Here's the drawing with two shaded views (mm, measured from the low corner). I have some questions. A direction names the side the tool comes from. Coordinates: 2 decimals unless noted, no trailing zeros. Order: outer loops, then holes, each group sorted by start corner. A loop starts at its lowest first (then second) coordinate and runs counter-clockwise, first axis right, second up. Notation, with made-up numbers: (15, 11) - (40, 11) arc R30 cw to (40, 43) - close; hole circle Ø6 at (-36.75, 8.25). An arc over 180 degrees is marked (long way). Answer as a JSON object with one key per item and string values. Group by question number.
(1) Imagine slicing it at C-C, the plane y = 6.25. Write out the boundary of the cut face in (x, z).
(2) Imagine slicing it at B-B, the plane x = 3. Write out the boundary of the cut face in (y, z), and give its area (3 significant figures).
(3) Will this pin go through, and if not, where does the flat tip stop? P1, Ø1.5, axis at y = 6, z = 4, coming from the +X side.
(4) Which directions (+Z, -Z, +X, -X, +Y, -Y) give clear straight access to the entire face, cutting with the end or side of a thin tool? Please do the marked faces 1, 2 and 3.
(5) Please list where these lines run through material, in increasing order: probe 1 along Z at (x, y) = (3.5, 0.75); probe 2 along Y at (x, z) = (2.7, 3.9); probe 3 along Z at (x, y) = (5, 2.25).
(6) Imagine slicing it at A-A, the plane y = 0.75. Write out the boundary of the cut face in (x, z).
(7) We'd pull the mould along Z, two halves only. Please class the marked faces 4, 5 and 6: pulls with the +Z half, pulls with the -Z half, needs draft (parallel to the pull), parting line crosses it, or undercut.
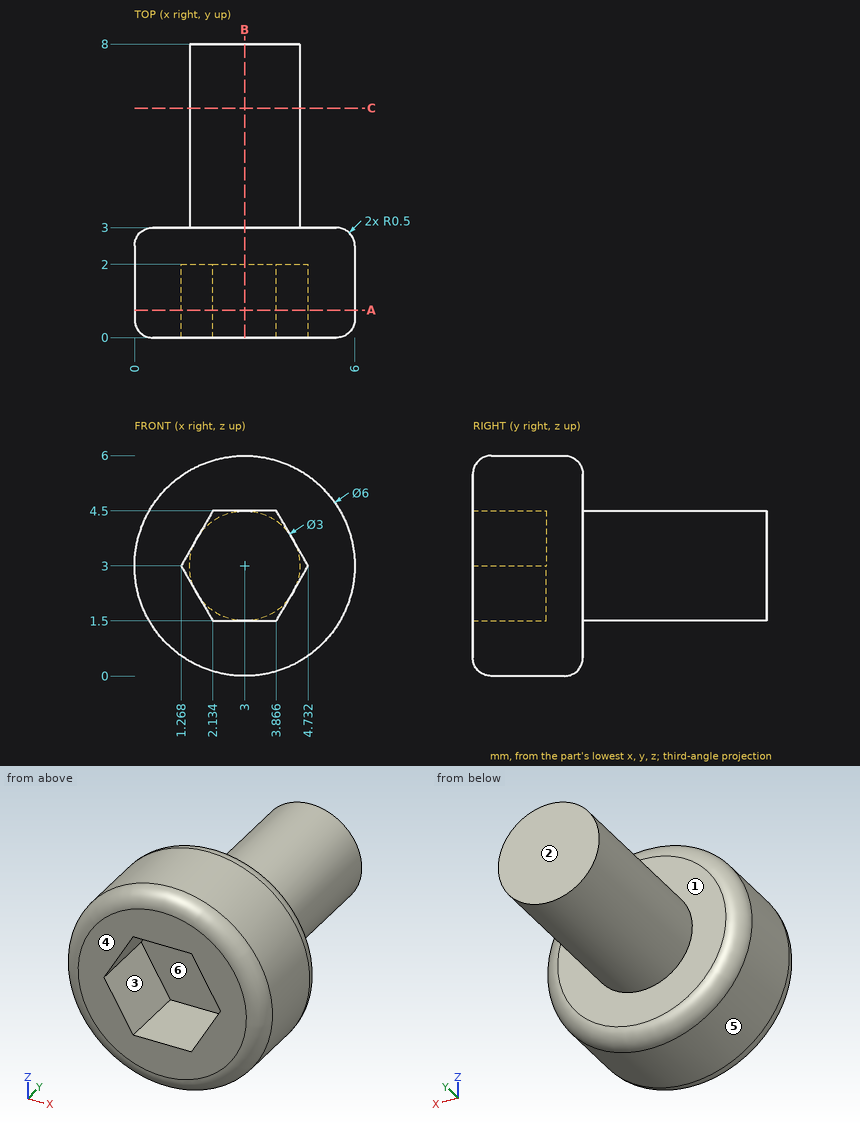
Result set:
{
 "1": {"outline": "circle Ø3 at (3, 3)"},
 "2": {"outline": "(0, 0.5) arc R0.5 ccw to (0.5, 0) - (2.5, 0) arc R0.5 ccw to (3, 0.5) - (3, 1.5) - (8, 1.5) - (8, 4.5) - (3, 4.5) - (3, 5.5) arc R0.5 ccw to (2.5, 6) - (0.5, 6) arc R0.5 ccw to (0, 5.5) - (0, 4.5) - (2, 4.5) - (2, 1.5) - (0, 1.5) - close", "area": "26.8 mm^2"},
 "3": {"P1": "stops at x = 4.48"},
 "4": {"face 1": "+Y", "face 2": "+Z, -Z, +X, -X, +Y", "face 3": "-Y"},
 "5": {"probe 1": "z = 0.04 to 1.5, 4.5 to 5.96", "probe 2": "y = 2 to 8", "probe 3": "z = 0.76 to 5.24"},
 "6": {"outline": "circle Ø6 at (3, 3); hole (1.27, 3) - (2.13, 1.5) - (3.87, 1.5) - (4.73, 3) - (3.87, 4.5) - (2.13, 4.5) - close"},
 "7": {"face 4": "needs draft", "face 5": "parting line crosses it", "face 6": "undercut"}
}
